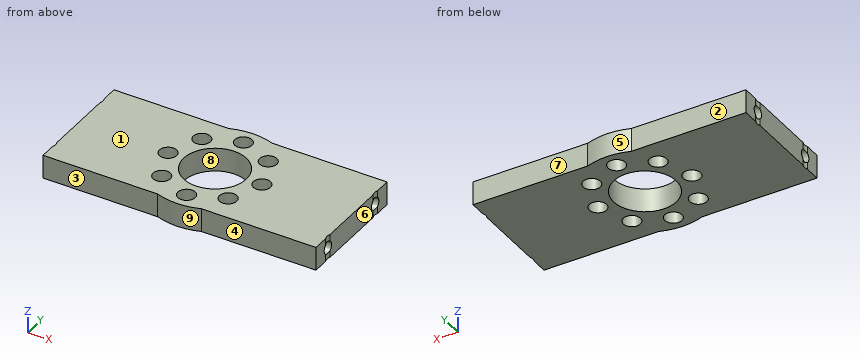
Autodesk Inventor part; units mm, degrees
ref_plane "YZ Plane" through (0, 0, 0) normal (1, 0, 0) x (0, 1, 0)
ref_plane "XZ Plane" through (0, 0, 0) normal (0, 1, 0) x (-1, 0, 0)
ref_plane "XY Plane" through (0, 0, 0) normal (0, 0, 1) x (1, 0, 0)
sketch "スケッチ1" plane through (0, 0, 0) normal (0, 0, 1) x (1, 0, 0)
  circle A0 centre (0, 0) radius 4
  circle A1 centre (0, 0) radius 8
  circle A2 centre (0, 0) radius 6 construction
  circle A3 centre (0, 6) radius 1.1
  circle A4 centre (-4.2426, 4.2426) radius 1.1
  circle A5 centre (-6, 0) radius 1.1
  circle A6 centre (-4.2426, -4.2426) radius 1.1
  circle A7 centre (0, -6) radius 1.1
  circle A8 centre (4.2426, -4.2426) radius 1.1
  circle A9 centre (6, 0) radius 1.1
  circle A10 centre (4.2426, 4.2426) radius 1.1
  line L0 (-17.45, -7.5) -> (17.45, -7.5)
  line L1 (17.45, -7.5) -> (17.45, 7.5)
  line L2 (17.45, 7.5) -> (-17.45, 7.5)
  line L3 (-17.45, 7.5) -> (-17.45, -7.5)
  line L4 (-17.45, -7.5) -> (17.45, 7.5) construction
  line L5 (17.45, -7.5) -> (-17.45, 7.5) construction
  point P0 (2.7839, 7.5)
  point P1 (-2.7839, 7.5)
  point P2 (2.7839, -7.5)
  point P3 (-2.7839, -7.5)
  dimension "d2" = 12
  dimension "d0" = 8
  dimension "d1" = 16
  dimension "d3" = 2.2
  dimension "d6" = 360
  dimension "d8" = 34.9
  dimension "d9" = 15
extrude "押し出し1" add sketch "スケッチ1" along normal blind 3
sketch "スケッチ2" plane through (17.45, -7.5, 0) normal (1, 0, 0) x (0, 0, -1)
  line L0 (0, 7.5) -> (-3, 7.5) construction
  line L1 (-3, 0) -> (-3, 15) construction
  line L2 (-1.5, 7.5) -> (-1.5, 15) construction
  line L3 (0, 15) -> (-3, 15) construction
  point P0 (-1.5, 12.5)
  point P1 (-1.5, 2.5)
  dimension "d12" = 5
hole "穴1" at (17.45, 5, 1.5) at (17.45, -5, 1.5) direction (-1, 0, 0) diameter 1.567 depth 4.5 tip angle 118
sketch "スケッチ3" plane through (-17.45, -7.5, 0) normal (-1, 0, 0) x (0, 0, 1)
  circle A0 centre (1.5, 2.5) radius 0.7835
  circle A1 centre (1.5, 12.5) radius 0.7835
  point P0 (0, 7.5)
  point P1 (1.5, 2.5)
  point P2 (1.5, 12.5)
hole "穴2" at (-17.45, -5, 1.5) at (-17.45, 5, 1.5) direction (1, 0, 0) diameter 1.567 depth 4.5 tip angle 118
sketch "スケッチ4" plane through (0, 0, 0) normal (0, 0, -1) x (-1, 0, 0)
  line L0 (17.45, -4.2165) -> (17.45, -5.7835)
  circle A0 centre (0, -6) radius 1.1
  line L1 (0, -6) -> (0, 0) construction
  circle A1 centre (18.45, -5) radius 1.1
  circle A2 centre (6, 0) radius 1.1 construction
  line L2 (0, 0) -> (6, 0) construction
  circle A3 centre (18.45, 5) radius 1.1
  line L3 (-17.45, -4.2165) -> (-17.45, -5.7835)
  circle A4 centre (-18.45, -5) radius 1.1
  circle A5 centre (-18.45, 5) radius 1.1
  point P0 (17.45, -5)
  point P1 (-17.45, -5)
  dimension "d27" = 2.2
  dimension "d28" = 1
extrude "押し出し2" cut sketch "スケッチ4" against normal blind 3 contours A1 L0 | L0 A1 | A3 | A4 L3 | L3 A4 | A5
properties part number "udeyi"
Verification items for the finished model (mm, model axes). Face numbers are marked on the shaded views. A direction names the side the tool comes from. Give positions to 0.01 mm unless a question says otherwise; leave off trailing zeros. Loops run counter-clockwise (first coordinate to the right, second up) from the corner with the lowest first, then second, coordinate; pieces in that order, holes last.
1. Section check B-B, the plane x = 0. Enter the section's corners in (y, z).
2. Section check D-D, the plane x = -6. Enter the section's corners in (y, z).
3. Section check A-A, the plane y = 0. Enter the section's corners in (x, z).
4. Thickness scan on line 1 (Y direction, x = 13.5, z = 1.4); line 2 (X direction, y = -4.25, z = 2); line 3 (Z direction, x = -16.25, y = 5). Record the ranges inside material, lowest first.
5. Go/stop test with flat-tipped pins: pin 1 Ø4 at (x, y) = (-4.5, 3) entering from -Z; pin 2 Ø0.9 at (x, z) = (-7.5, 1.5) entering from -Y; pin 3 Ø1.4 at (y, z) = (5, 1.5) entering from +X; pin 4 Ø1.4 at (y, z) = (5, 1.5) entering from -X. Record where each tip stops, or that it passes through.
6. Mould release check, pull along Y, two halves, no side actions. Record for the marked faces 6, 7, 8 and 9: released by +Y, released by -Y, zero draft, split by the parting line, or undercut.
7. Section check C-C, the plane x = 14.5. Enter the section's corners in (y, z).
8. Set-up check for the marked faces 1, 2, 3, 4 and 5: record each of +Z, -Z, +X, -X, +Y, -Y from which the full face is reachable in a straight line by a thin tool's end or side.
Geometry says:
1. outline: (-8, 0) - (-7.1, 0) - (-7.1, 3) - (-8, 3) - close; (-4.9, 0) - (-4, 0) - (-4, 3) - (-4.9, 3) - close; (4, 0) - (4.9, 0) - (4.9, 3) - (4, 3) - close; (7.1, 0) - (8, 0) - (8, 3) - (7.1, 3) - close
2. outline: (-7.5, 0) - (-1.1, 0) - (-1.1, 3) - (-7.5, 3) - close; (1.1, 0) - (7.5, 0) - (7.5, 3) - (1.1, 3) - close
3. outline: (-17.45, 0) - (-7.1, 0) - (-7.1, 3) - (-17.45, 3) - close; (-4.9, 0) - (-4, 0) - (-4, 3) - (-4.9, 3) - close; (4, 0) - (4.9, 0) - (4.9, 3) - (4, 3) - close; (7.1, 0) - (17.45, 0) - (17.45, 3) - (7.1, 3) - close
4. line 1: y = -7.5 to -5.78, -4.22 to 4.22, 5.78 to 7.5
4. line 2: x = -17.45 to -5.34, -3.14 to 3.14, 5.34 to 17.45
4. line 3: z = 0 to 0.72, 2.28 to 3
5. pin 1: stops at z = 0
5. pin 2: stops at y = -7.5
5. pin 3: stops at x = 12.9
5. pin 4: stops at x = -12.9
6. face 6: zero draft
6. face 7: released by +Y
6. face 8: undercut
6. face 9: released by -Y
7. outline: (-7.5, 0) - (7.5, 0) - (7.5, 3) - (-7.5, 3) - close; hole circle Ø1.57 at (-5, 1.5); hole circle Ø1.57 at (5, 1.5)
8. face 1: +Z, +X, -X, +Y, -Y
8. face 2: +Z, -Z, -X, +Y
8. face 3: +Z, -Z, -X, -Y
8. face 4: +Z, -Z, +X, -Y
8. face 5: +Z, -Z, +Y
